CAD build for the part. Positions are in the model's coordinates, mm. Face numbers are marked on the shaded views. Coordinates: 2 decimals unless noted, no trailing zeros. Loops run counter-clockwise (first coordinate to the right, second up) from the corner with the lowest first, then second, coordinate; pieces in that order, holes last. Notation, with made-up numbers: (-22, 42.25) -> (2, 42.25) arc R23 ccw to (2, 79.25) -> close; hole circle Ø2 at (52, -3.5). An arc over 180 degrees is marked (long way). Answer as a JSON object with one key per item and string values. Group by question number.
from build123d import *

# Parameters (mm, degrees)
BOSS_EXTRUDE1_DEPTH = 80
SKETCH2_R           = 6.272806616
CUT_EXTRUDE1_DEPTH  = 500


with BuildPart() as part:
    # Sketch1 → Boss-Extrude1 (new body)
    with BuildSketch(Plane.XY):
        Polygon((125, 0), (-125, 0), (-125, 83), (-122, 83), (-122, 3), (122, 3), (122, 83), (125, 83), align=None)
    extrude(amount=BOSS_EXTRUDE1_DEPTH)

    # Sketch2 → Cut-Extrude1 (cut)
    with BuildSketch(Plane.ZY.offset(125)):
        with Locations((40, 67.971243919)):
            Circle(SKETCH2_R)
    extrude(amount=-CUT_EXTRUDE1_DEPTH, mode=Mode.SUBTRACT)


solid = part.part
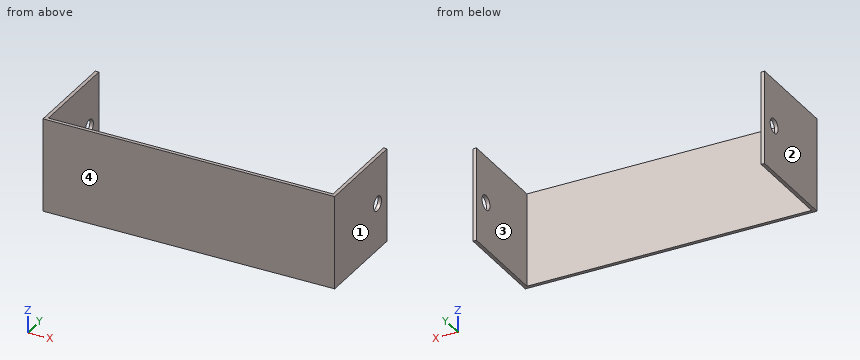
Item 1: Pull direction X, two halves, no side cores. Call the marked faces 1, 2, 3 and 4: +X half, -X half, draft (parallel to the pull), parting line (faces both ways), or undercut.
Item 2: Band-saw the part on B-B, the plane y = 53.5. List the corners of the cut face in (x, z).
Item 3: Band-saw the part on C-C, the plane z = 68. List the corners of the cut face in (x, y), and give its area (3 significant figures).
Item 4: Band-saw the part on A-A, the plane z = 40. List the corners of the cut face in (x, y).
Item 5: Band-saw the part on D-D, the plane x = -78. List the corners of the cut face in (y, z), and give its area (3 significant figures).
Item 6: Flat gauge pin, fed straight in: P1, Ø3, axis at x = 26.5, z = 24, coming from the +Y side. Where does the tip first touch, or does it go through?
Item 7: Drill centre lines: L1, parallel to X at y = 47.5, z = 27; L2, parallel to Y at x = -123.4, z = 40; L3, parallel to Y at x = -61, z = 7. Where is each one in solid material? Low to high.
Reply:
{
 "1": {"face 1": "+X half", "face 2": "-X half", "face 3": "undercut", "face 4": "draft"},
 "2": {"outline": "(-125, 0) -> (-122, 0) -> (-122, 80) -> (-125, 80) -> close; (122, 0) -> (125, 0) -> (125, 80) -> (122, 80) -> close"},
 "3": {"outline": "(-125, 0) -> (125, 0) -> (125, 83) -> (122, 83) -> (122, 3) -> (-122, 3) -> (-122, 83) -> (-125, 83) -> close", "area": "1,230 mm²"},
 "4": {"outline": "(-125, 0) -> (125, 0) -> (125, 61.7) -> (122, 61.7) -> (122, 3) -> (-122, 3) -> (-122, 61.7) -> (-125, 61.7) -> close; (-125, 74.24) -> (-122, 74.24) -> (-122, 83) -> (-125, 83) -> close; (122, 74.24) -> (125, 74.24) -> (125, 83) -> (122, 83) -> close"},
 "5": {"outline": "(0, 0) -> (3, 0) -> (3, 80) -> (0, 80) -> close", "area": "240 mm²"},
 "6": {"P1": "y = 3"},
 "7": {"L1": "-125 to -122, 122 to 125", "L2": "0 to 61.7, 74.24 to 83", "L3": "0 to 3"}
}
